Verification items for the finished model (mm, model axes). Round coordinates to 2 decimals unless told otherwise and drop trailing zeros. Write each loop counter-clockwise with the first axis right and the second up, starting at its lowest first coordinate (ties: lowest second). Pieces come first, ordered by that corner, then holes. Notation, with made-up numbers: M 75.25,73 L 132.25,73 A6 cw 132.25,80 Z; hole C 75,7.25 d8. An arc over 180 degrees is marked long. One line per item, written item: value. Start each with the question number.
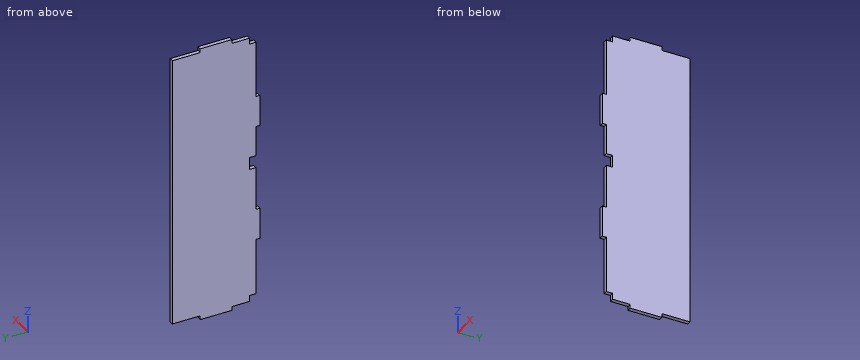
from build123d import *

# Parameters (mm, degrees)
BOSS_EXTRUDE1_DEPTH = 3.175
SKETCH2_W           = 222.25
SKETCH2_H           = 3.175
CUT_EXTRUDE1_DEPTH  = 4.175
SKETCH3_W           = 5
SKETCH3_H           = 5
SKETCH3_W_2         = 10
CUT_EXTRUDE2_DEPTH  = 10


with BuildPart() as part:
    # Sketch1 → Boss-Extrude1 (new body)
    with BuildSketch(Plane(origin=(0, 0, 0), x_dir=(0, 0, -1), z_dir=(1, 0, 0))):
        Polygon((-105.784096482, 33.834012461), (-105.784096482, 8.434012461), (-108.959096482, 8.434012461), (-108.959096482, -16.965987539), (-105.784096482, -16.965987539), (-105.784096482, -36.015987539), (-54.984096482, -36.015987539), (-54.984096482, -39.190987539), (-29.584096482, -39.190987539), (-29.584096482, -36.015987539), (40.265903518, -36.015987539), (40.265903518, -39.190987539), (65.665903518, -39.190987539), (65.665903518, -36.015987539), (116.465903518, -36.015987539), (116.465903518, -16.965987539), (119.640903518, -16.965987539), (119.640903518, 8.434012461), (116.465903518, 8.434012461), (116.465903518, 33.834012461), align=None)
    extrude(amount=BOSS_EXTRUDE1_DEPTH)

    # Sketch2 → Cut-Extrude1 (cut, through all)
    with BuildSketch(Plane(origin=(3.175, 0, 0), x_dir=(0, 0, -1), z_dir=(1, 0, 0))):
        with Locations((5.340903518, 32.246512461)):
            Rectangle(SKETCH2_W, SKETCH2_H)
    extrude(amount=-CUT_EXTRUDE1_DEPTH, mode=Mode.SUBTRACT)

    # Sketch3 → Cut-Extrude2 (cut)
    with BuildSketch(Plane(origin=(3.175, 0, 0), x_dir=(0, 0, -1), z_dir=(1, 0, 0))):
        with Locations((-103.284096482, -33.515987539)):
            Rectangle(SKETCH3_W, SKETCH3_H)
        with Locations((113.965903518, -33.515987539)):
            Rectangle(SKETCH3_W, SKETCH3_H)
        with Locations((0, -33.515987539)):
            Rectangle(SKETCH3_W_2, SKETCH3_H)
    extrude(amount=-CUT_EXTRUDE2_DEPTH, mode=Mode.SUBTRACT)


solid = part.part
1) Thickness scan on line 1 (Y direction, x = 1.25, z = 6.5); line 2 (Z direction, x = 2.9, y = 15.5). Record the ranges inside material, lowest first.
2) Gauge pin test, flat ends, axial feed: pin 1 Ø1 at (x, z) = (1.5, -118) entering from +Y; pin 2 Ø1 at (x, y) = (1.5, -37.5) entering from -Z; pin 3 Ø1 at (x, z) = (2.5, 107) entering from -Y. Record the tip position at first contact, or that the pin passes through.
3) Cross-section at A-A (x = 1.15). Record the boundary of the cut face in (y, z).
4) Cross-section at B-B (y = -25). Record the boundary of the cut face in (x, z) (3 decimals), then the cut area to 3 significant figures.
5) Cross-section at C-C (z = 78.5). Record the boundary of the cut face in (x, y) (3 decimals), then the cut area to 3 significant figures.
Results below:
1. line 1: y = -36.02 to 30.66
1. line 2: z = -116.47 to 105.78
2. pin 1: stops at y = 8.43
2. pin 2: stops at z = -65.67
2. pin 3: stops at y = -16.97
3. outline: M -39.19,-65.67 L -36.02,-65.67 L -36.02,-111.47 L -31.02,-111.47 L -31.02,-116.47 L -16.97,-116.47 L -16.97,-119.64 L 8.43,-119.64 L 8.43,-116.47 L 30.66,-116.47 L 30.66,105.78 L 8.43,105.78 L 8.43,108.96 L -16.97,108.96 L -16.97,105.78 L -31.02,105.78 L -31.02,100.78 L -36.02,100.78 L -36.02,54.98 L -39.19,54.98 L -39.19,29.58 L -36.02,29.58 L -36.02,5 L -31.02,5 L -31.02,-5 L -36.02,-5 L -36.02,-40.27 L -39.19,-40.27 Z
4. outline: M 0,-116.466 L 3.175,-116.466 L 3.175,105.784 L 0,105.784 Z
4. area: 706 mm²
5. outline: M 0,-36.016 L 3.175,-36.016 L 3.175,30.659 L 0,30.659 Z
5. area: 212 mm²
